from build123d import *

# Parameters (mm, degrees)
F0_R     = 16.5
F1_DEPTH = 2.54
F2_R     = 12.7
F3_DEPTH = 3.175
F4_R     = 2.53999
F5_R     = 0.79375


# Not quite as in the source:
# - a fillet or chamfer is up to 0.001 mm smaller than in the source, because OpenCascade refuses the exact size


with BuildPart() as f1:
    # F0 (on Top) → F1 (new body)
    with BuildSketch(Plane.XY):
        Circle(F0_R)
    extrude(amount=F1_DEPTH)

    # F2 (on face) → F3 (join)
    with BuildSketch(Plane.XY.offset(2.54)):
        Circle(F2_R)
    extrude(amount=F3_DEPTH)

    # F4 (radius 2.54 in the source; OpenCascade refuses exactly that, so slightly less here)
    f4_edges = [f1.edges().sort_by_distance(p)[0] for p in [
        (-16.5, 0, 2.54),
    ]]
    fillet(f4_edges, radius=F4_R)

    # F5
    f5_edges = [f1.edges().sort_by_distance(p)[0] for p in [
        (-12.7, 0, 5.715),
    ]]
    fillet(f5_edges, radius=F5_R)


solid = f1.part
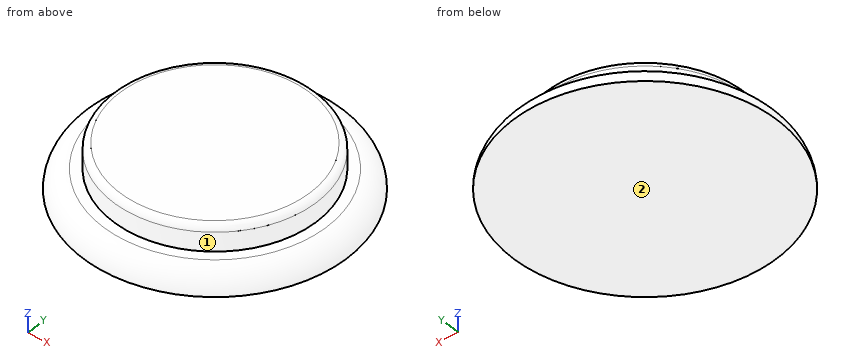
Here's how the part is built. I have some questions about the finished solid (model axes, mm). Face numbers are marked on the shaded views. A direction names the side the tool comes from. Give positions to 0.01 mm unless a question says otherwise; leave off trailing zeros. Order: outer loops, then holes, each group sorted by start corner. A loop starts at its lowest first (then second) coordinate and runs counter-clockwise, first axis right, second up. Notation, with made-up numbers: M 37,-20 L 61,-20 A19 ccw 61,-16 Z; hole C 56,-30.75 d5. An arc over 180 degrees is marked long. Answer as a JSON object with one key per item and string values. Group by question number.
1) Please list where these lines run through material, in increasing order: L1, parallel to Y at x = -1.5, z = 0.8; L2, parallel to Y at x = 10.5, z = 0.5. Write a range as [from, to].
2) On a 3-axis mill with a long thin cutter (end or side, diameter ignored), from which of +Z, -Z, +X, -X, +Y, -Y can I reach the whole of each face in a straight line? I mean the marked faces 1 and 2. Say none if no direction works.
3) Suppose I cut it at C-C, the plane z = 1.45. Write out the boundary of the cut face in (x, y), plus the area to 3 significant figures.
4) I'm going to push flat-ended pins straight in: pin 1 Ø3 at (x, z) = (5.5, 4.5) entering from -Y; pin 2 Ø2 at (y, z) = (12.5, 2) entering from -X; pin 3 Ø1 at (y, z) = (6.5, 3.5) entering from -X. Where does each tip first touch, or does it pass through?
Results found:
{
 "1": {"L1": "[-16.3, 16.3]", "L2": "[-12.66, 12.66]"},
 "2": {"face 1": "+Z", "face 2": "-Z, +X, -X, +Y, -Y"},
 "3": {"outline": "C 0,0 d32.09", "area": "809 mm²"},
 "4": {"pin 1": "y = -12.05", "pin 2": "x = -11.03", "pin 3": "x = -11.19"}
}
